from build123d import *

# Parameters (mm, degrees)
SKETCH_1_R          = 3
SKETCH_1_R_2        = 1.6
EXTRUDE_1_DEPTH     = 4
FILLET_1_R          = 3
FILLET_2_R          = 25
SKETCH_2_R          = 1.6
CUT_EXTRUDE_1_DEPTH = 10
SKETCH_3_R          = 3
CUT_EXTRUDE_2_DEPTH = 10
EXTRUDE_2_DEPTH     = 4
FILLET_3_R          = 5
FILLET_4_R          = 1
SKETCH_5_R          = 1.6
CUT_EXTRUDE_3_DEPTH = 10


with BuildPart() as part:
    # ｽｹｯﾁ1 → ﾎﾞｽ - 押し出し1 (new body)
    with BuildSketch(Plane.XY):
        Polygon((-32, -10.4), (-32, -31), (27, -31), (27, 54), (-32, 54), (-32, 35.9), (20.65, 35.9), (20.65, 15.1), (-32, 15.1), (-32, 10.4), align=None)
        with Locations((10.2, -19.5)):
            Circle(SKETCH_1_R, mode=Mode.SUBTRACT)
        with Locations((24.3, 20.55)):
            Circle(SKETCH_1_R_2, mode=Mode.SUBTRACT)
        with Locations((24.3, 30.45)):
            Circle(SKETCH_1_R_2, mode=Mode.SUBTRACT)
        with Locations((10.2, 42.5)):
            Circle(SKETCH_1_R, mode=Mode.SUBTRACT)
    extrude(amount=EXTRUDE_1_DEPTH)

    # ﾌｨﾚｯﾄ1
    fillet_1_edges = [part.edges().sort_by_distance(p)[0] for p in [
        (-32, 54, 2),
        (-32, -31, 2),
    ]]
    fillet(fillet_1_edges, radius=FILLET_1_R)

    # ﾌｨﾚｯﾄ2
    fillet_2_edges = [part.edges().sort_by_distance(p)[0] for p in [
        (27, 54, 2),
        (27, -31, 2),
    ]]
    fillet(fillet_2_edges, radius=FILLET_2_R)

    # ｽｹｯﾁ2 → ｶｯﾄ - 押し出し1 (cut)
    with BuildSketch(Plane(origin=(0, 0, 0), x_dir=(-1, 0, 0), z_dir=(0, 0, -1))):
        with Locations((27, 49)):
            Circle(SKETCH_2_R)
        with Locations((27, -26)):
            Circle(SKETCH_2_R)
    extrude(amount=-CUT_EXTRUDE_1_DEPTH, mode=Mode.SUBTRACT)

    # ｽｹｯﾁ3 → ｶｯﾄ - 押し出し2 (cut)
    with BuildSketch(Plane(origin=(0, 0, 0), x_dir=(-1, 0, 0), z_dir=(0, 0, -1))):
        with Locations((-10.2, -2.5)):
            Circle(SKETCH_3_R)
    extrude(amount=-CUT_EXTRUDE_2_DEPTH, mode=Mode.SUBTRACT)

    # ｽｹｯﾁ4 → ﾎﾞｽ - 押し出し2 (add)
    with BuildSketch(Plane(origin=(0, 0, 0), x_dir=(-1, 0, 0), z_dir=(0, 0, -1))):
        Polygon((-27, 19.5), (-43.945270358, 19.5), (-38.364198183, 11.5), (-44.023561215, 3.5), (-27, 3.5), align=None)
    extrude(amount=-EXTRUDE_2_DEPTH)

    # ﾌｨﾚｯﾄ3
    fillet_3_edges = [part.edges().sort_by_distance(p)[0] for p in [
        (27, 19.5, 2),
        (27, 3.5, 2),
    ]]
    fillet(fillet_3_edges, radius=FILLET_3_R)

    # ﾌｨﾚｯﾄ4
    fillet_4_edges = [part.edges().sort_by_distance(p)[0] for p in [
        (38.364198183, 11.5, 2),
    ]]
    fillet(fillet_4_edges, radius=FILLET_4_R)

    # ｽｹｯﾁ5 → ｶｯﾄ - 押し出し3 (cut)
    with BuildSketch(Plane.XY.offset(4)):
        with Locations((-2, -26)):
            Circle(SKETCH_5_R)
        with Locations((-2, 49)):
            Circle(SKETCH_5_R)
    extrude(amount=-CUT_EXTRUDE_3_DEPTH, mode=Mode.SUBTRACT)


solid = part.part
Here's how the part is built. I have some questions about the finished solid (model axes, mm). A direction names the side the tool comes from. Round coordinates to 2 decimals unless told otherwise and drop trailing zeros. Loops run counter-clockwise (first coordinate to the right, second up) from the corner with the lowest first, then second, coordinate; pieces in that order, holes last. Notation, with made-up numbers: (36, -31.75) -> (42, -31.75) arc R8 cw to (42, -20.75) -> close; hole circle Ø9 at (49, 15). An arc over 180 degrees is marked (long way). Write each question's results on one line, items separated by ' | '.
(1) If we section it at D-D, the plane x = 12: List the corners of the cut face in (y, z) for me.
Worked answers:
outline: (-28.91, 0) -> (-21.9, 0) -> (-21.9, 4) -> (-28.91, 4) -> close; (-17.1, 0) -> (-4.9, 0) -> (-4.9, 4) -> (-17.1, 4) -> close; (-0.1, 0) -> (15.1, 0) -> (15.1, 4) -> (-0.1, 4) -> close; (35.9, 0) -> (40.1, 0) -> (40.1, 4) -> (35.9, 4) -> close; (44.9, 0) -> (51.91, 0) -> (51.91, 4) -> (44.9, 4) -> close
(2) If we section it at A-A, the plane y = -2.5: List the corners of the cut face in (x, z) for me, then the cut area to 3 significant figures.
Worked answers:
outline: (-32, 0) -> (7.2, 0) -> (7.2, 4) -> (-32, 4) -> close; (13.2, 0) -> (27, 0) -> (27, 4) -> (13.2, 4) -> close | area: 212 mm2
(3) If we section it at B-B, the plane x = -27: List the corners of the cut face in (y, z) for me, then the cut area to 3 significant figures.
Worked answers:
outline: (-31, 0) -> (-27.6, 0) -> (-27.6, 4) -> (-31, 4) -> close; (-24.4, 0) -> (15.1, 0) -> (15.1, 4) -> (-24.4, 4) -> close; (35.9, 0) -> (47.4, 0) -> (47.4, 4) -> (35.9, 4) -> close; (50.6, 0) -> (54, 0) -> (54, 4) -> (50.6, 4) -> close | area: 231 mm2
(4) If I drill on L1, parallel to Y at x = -27, z = 2.25; L2, parallel to X at y = -25.5, z = 0.6; L3, parallel to Y at x = -8.5, z = 2, over which ranges is the centre line in solid material (lowest first)?
Worked answers:
L1: -31 to -27.6, -24.4 to 15.1, 35.9 to 47.4, 50.6 to 54 | L2: -32 to -28.52, -25.48 to -3.52, -0.48 to 17.64 | L3: -31 to 15.1, 35.9 to 54
(5) For P1, Ø5, axis at x = 10.2, y = -19.5, coming from the +Z side; P2, Ø2, axis at y = 27, z = 2, coming from the +X side, each with a flat end and sliding along its axis, tell me the tip position at first contact or that it passes through.
Worked answers:
P1: through | P2: x = 27
(6) If we section it at C-C, the plane z = 2.1: Give the number of separate pieces and of enclosed holes in the cut face, then the cut area to 3 significant figures.
Worked answers:
separate pieces: 1 | enclosed holes: 9 | area: 3,750 mm2
(7) For faces 1 (the face through (27, 27, 2)), 2 (the face through (-13, 54, 2)), 3 (the face through (27, -4, 2)), which set-ups out of +Z, -Z, +X, -X, +Y, -Y let a thin tool reach every point of the face, with its end or its side?
Worked answers:
face 1: +Z, -Z, +X, +Y | face 2: +Z, -Z, +X, -X, +Y | face 3: +Z, -Z, +X, -Y
(8) We'd pull the mould along X, two halves only. Please class faces 4 (the face through (-6, 35.9, 2)), 5 (the face through (-31.1, -30.14, 2.03)), 6 (the face through (-1.14, 50.35, 2.03)), 7 (the face through (41.36, 7.265, 1.972)): released by +X, released by -X, zero draft, split by the parting line, or undercut.
Worked answers:
face 4: zero draft | face 5: released by -X | face 6: undercut | face 7: released by +X
